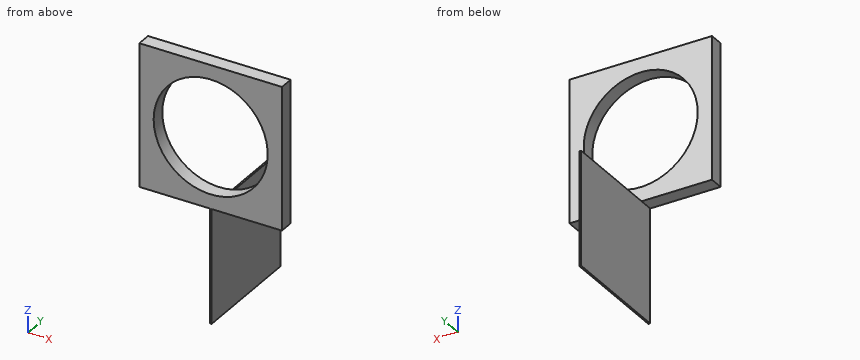
from build123d import *

# Parameters (mm, degrees)
F0_W     = 127
F0_H     = 127
F1_DEPTH = 12.7
F3_D     = 101.6
F4_W     = 1.5875
F4_H     = 88.9
F4_H_2   = 12.7
F5_DEPTH = 101.6


with BuildPart() as f1:
    # F0 (on Front) → F1 (new body)
    with BuildSketch(Plane.XZ):
        with Locations((-63.5, 63.5)):
            Rectangle(F0_W, F0_H)
    extrude(amount=F1_DEPTH)

    # F3 (through all)
    with Locations(Plane.XZ.offset(12.7)):
        with Locations((-63.5, 63.5)):
            Hole(F3_D / 2)

    # F4 (on face) → F5 (join)
    with BuildSketch(Plane(origin=(0, 0, 0), x_dir=(1, 0, 0), z_dir=(0, 0, -1))):
        with Locations((-63.5, -44.45)):
            Rectangle(F4_W, F4_H)
        with Locations((-63.5, 6.35)):
            Rectangle(F4_W, F4_H_2)
    extrude(amount=F5_DEPTH)


solid = f1.part
Input: part model. Units: mm. Frame: model coordinates. Give positions to 0.01 mm unless a question says otherwise; leave off trailing zeros. Write each loop counter-clockwise with the first axis right and the second up, starting at its lowest first coordinate (ties: lowest second). Pieces come first, ordered by that corner, then holes. Notation, with made-up numbers: M 87.25,77.25 L 97.25,77.25 A24 ccw 97.25,112.25 Z; hole C 86.25,89.5 d3. An arc over 180 degrees is marked long. Use one line per item in the form item = value.
1. First-contact query: P1, Ø4, axis at x = -24, y = -6.5, coming from the -Z side; P2, Ø2, axis at y = 67, z = -1.5, coming from the -X side; P3, Ø0.8, axis at x = -63.5, y = 29.5, coming from the +Z side; P4, Ø10, axis at x = -86.5, z = -7, coming from the -Y side. Flat tips, straight axial feed; report the tip coordinate or a pass-through.
Outcome:
P1 = 0
P2 = -64.29
P3 = 0
P4 = through
2. Cut plane D-D on z = -12. Return loops of the section in (x, y), and give its area (3 significant figures).
Outcome:
outline = M -64.29,-12.7 L -62.71,-12.7 L -62.71,88.9 L -64.29,88.9 Z
area = 161 mm²
3. Cut plane C-C on y = 47. Return loops of the section in (x, z).
Outcome:
outline = M -64.29,-101.6 L -62.71,-101.6 L -62.71,0 L -64.29,0 Z
4. Ray query, L1, parallel to Z at x = -63.5, y = -5; L2, parallel to X at y = 82.5, z = -39.5; L3, parallel to Y at x = -51, z = 8. Return the intervals inside material, ascending.
Outcome:
L1 = -101.6 to 12.7, 114.3 to 127
L2 = -64.29 to -62.71
L3 = -12.7 to 0
5. Cut plane A-A on z = 63.5. Return loops of the section in (x, y).
Outcome:
outline = M -127,-12.7 L -114.3,-12.7 L -114.3,0 L -127,0 Z; M -12.7,-12.7 L 0,-12.7 L 0,0 L -12.7,0 Z
6. Cut plane B-B on x = -20. Return loops of the section in (y, z).
Outcome:
outline = M -12.7,0 L 0,0 L 0,37.26 L -12.7,37.26 Z; M -12.7,89.74 L 0,89.74 L 0,127 L -12.7,127 Z
